Read the model definition and answer for the solid it produces. Units are mm, in the model's axes. A direction names the side the tool comes from. Coordinates: 2 decimals unless noted, no trailing zeros. Write each loop counter-clockwise with the first axis right and the second up, starting at its lowest first coordinate (ties: lowest second). Pieces come first, ordered by that corner, then holes.
(1) Straight lines are drawn through the part: line 1 along Y through (x, z) = (9, -5); line 2 along Z through (x, y) = (16.5, 0); line 3 along X through (y, z) = (-2.95, 0). For each, find the intervals that lie inside material, in ascending order.
(2) Determine the mould class of faces 5 (the cylindrical face through (10.074, -5.014, 0.404)), 6 (the cylindrical face through (14.79, 1.23, 6.14)), 7 (the flat face through (15, 6, 0)) for opening direction Y: pulls with the +Y half, pulls with the -Y half, needs draft (parallel to the pull), parting line crosses it, or undercut.
(3) The part is cut by section D-D, the plane z = -10.05. Determine the outline of the cut face in (x, y).
(4) The part is cut by section B-B, the plane y = 0. Determine the outline of the cut face in (x, z).
(5) The part is cut by section C-C, the plane x = 7. Determine the outline of the cut face in (y, z), and give its area (3 significant figures).
(6) Which of the six approach directions +Z, -Z, +X, -X, +Y, -Y give full straight-line access (tool end or side, diameter ignored) to faces 1 (the flat face through (20, -12, 14.15)), 2 (the flat face through (24, -14, 15)), 3 (the flat face through (9, 1, 0)), 4 (the flat face through (5.7, -4, -1.3))?
(7) The part is cut by section A-A, the plane z = 0. Determine the outline of the cut face in (x, y), and give its area (3 significant figures).
(8) Given pin 1 (6 mm diameter, centred on x = 4, z = 4, fed in from -Y); pin 2 (1 mm diameter, centred on y = 0, z = -15, fed in from -X); pin 3 (3 mm diameter, centred on x = 6.5, z = 1, fed in from -Y), each flat-ended and moving along its own axis, determine where each tip first touches the part or whether it passes through.
```python
from build123d import *

# Parameters (mm, degrees)
CROQUIS1_W              = 32.1
CROQUIS1_H              = 12
CROQUIS1_R              = 4.1
SALIENTE_EXTRUIR1_DEPTH = 30
CROQUIS2_W              = 15
CROQUIS2_H              = 2
CORTAR_EXTRUIR2_DEPTH   = 33
CROQUIS4_R              = 1.65
CORTAR_EXTRUIR3_DEPTH   = 12
CROQUIS5_R              = 3.1
CORTAR_EXTRUIR4_DEPTH   = 2
SALIENTE_EXTRUIR2_DEPTH = 16
REDONDEO1_R             = 5
REDONDEO2_R             = 5
REDONDEO3_RADIUS        = 4.002255821
REDONDEO3_LENGTH        = 1.9


with BuildPart() as part:
    # Croquis1 → Saliente-Extruir1 (new body)
    with BuildSketch(Plane(origin=(0, 0, 0), x_dir=(0, 0, -1), z_dir=(1, 0, 0))):
        Rectangle(CROQUIS1_W, CROQUIS1_H)
        with Locations((-10.05, 0)):
            Circle(CROQUIS1_R, mode=Mode.SUBTRACT)
        with Locations((10.05, 0)):
            Circle(CROQUIS1_R, mode=Mode.SUBTRACT)
    extrude(amount=SALIENTE_EXTRUIR1_DEPTH)

    # Croquis2 → Cortar-Extruir2 (cut)
    with BuildSketch(Plane.XY.offset(16.05)):
        with Locations((7.5, 0)):
            Rectangle(CROQUIS2_W, CROQUIS2_H)
    extrude(amount=-CORTAR_EXTRUIR2_DEPTH, mode=Mode.SUBTRACT)

    # Croquis4 → Cortar-Extruir3 (cut)
    with BuildSketch(Plane(origin=(0, 6, 0), x_dir=(1, 0, 0), z_dir=(0, 1, 0))):
        with Locations(Location((7, 0, 0), (0, 0, 270))):
            Circle(CROQUIS4_R)
    extrude(amount=-CORTAR_EXTRUIR3_DEPTH, mode=Mode.SUBTRACT)

    # Croquis5 → Cortar-Extruir4 (cut)
    with BuildSketch(Plane.XZ.offset(6)):
        with Locations(Location((7, 0, 0), (0, 0, 270))):
            Circle(CROQUIS5_R)
    extrude(amount=-CORTAR_EXTRUIR4_DEPTH, mode=Mode.SUBTRACT)

    # Croquis7 → Saliente-Extruir2 (add)
    with BuildSketch(Plane.XZ.offset(6)):
        Polygon((20, 14.15), (24, 14.15), (24, 16.05), (15.995488358, 16.05), (15.995488358, 14.15), align=None)
    extrude(amount=SALIENTE_EXTRUIR2_DEPTH)

    # Redondeo1
    redondeo1_edges = [part.edges().sort_by_distance(p)[0] for p in [
        (15.995488358, -6, 15.1),
    ]]
    fillet(redondeo1_edges, radius=REDONDEO1_R)

    # Redondeo2
    redondeo2_edges = [part.edges().sort_by_distance(p)[0] for p in [
        (24, -6, 15.1),
    ]]
    fillet(redondeo2_edges, radius=REDONDEO2_R)

    # Redondeo3: full round fillet: the end face becomes a half cylinder, R = half its width
    redondeo3_face = Plane((19.997744179, -22, 15.1), x_dir=(0, 0, 1), z_dir=(0, -1, 0))  # on the end face: x along it, z out of the body
    redondeo3_slab = redondeo3_face.offset(-REDONDEO3_RADIUS / 2) * Box(REDONDEO3_LENGTH, 2 * REDONDEO3_RADIUS, REDONDEO3_RADIUS, mode=Mode.PRIVATE)  # the body's end, R deep
    redondeo3_round = Plane((19.997744179, -17.997744179, 15.1), x_dir=(0, -1, 0), z_dir=(0, 0, 1)) * Cylinder(REDONDEO3_RADIUS, REDONDEO3_LENGTH, mode=Mode.PRIVATE)  # its axis R under the face
    add(redondeo3_slab - redondeo3_round, mode=Mode.SUBTRACT)


solid = part.part
```
Computed:
1. line 1: y = -6 to -1, 1 to 6
1. line 2: z = -16.05 to -14.15, -5.95 to 5.95, 14.15 to 16.05
1. line 3: x = 0 to 5.35, 8.65 to 30
2. face 5: needs draft
2. face 6: undercut
2. face 7: pulls with the +Y half
3. outline: (0, -6) - (30, -6) - (30, -4.1) - (0, -4.1) - close; (0, 4.1) - (30, 4.1) - (30, 6) - (0, 6) - close
4. outline: (15, -16.05) - (30, -16.05) - (30, -14.15) - (15, -14.15) - close; (15, -5.95) - (30, -5.95) - (30, 5.95) - (15, 5.95) - close; (15, 14.15) - (30, 14.15) - (30, 16.05) - (15, 16.05) - close
5. outline: (-6, -16.05) - (-1, -16.05) - (-1, -14.03) arc R4.1 cw to (-1, -6.07) - (-1, -1.65) - (-4, -1.65) - (-4, -3.1) - (-6, -3.1) - close; (-6, 3.1) - (-4, 3.1) - (-4, 1.65) - (-1, 1.65) - (-1, 6.07) arc R4.1 cw to (-1, 14.03) - (-1, 16.05) - (-6, 16.05) - close; (1, -16.05) - (6, -16.05) - (6, -1.65) - (1, -1.65) - (1, -6.07) arc R4.1 cw to (1, -14.03) - close; (1, 1.65) - (6, 1.65) - (6, 16.05) - (1, 16.05) - (1, 14.03) arc R4.1 cw to (1, 6.07) - close
5. area: 209 mm2
6. face 1: -Z, +X, -X, -Y
6. face 2: +Z, -Z, +X, -Y
6. face 3: +Z, -Z, -X
6. face 4: -Y
7. outline: (0, -6) - (3.9, -6) - (3.9, -4) - (5.35, -4) - (5.35, -1) - (0, -1) - close; (0, 1) - (5.35, 1) - (5.35, 6) - (0, 6) - close; (8.65, -4) - (10.1, -4) - (10.1, -6) - (30, -6) - (30, 6) - (8.65, 6) - (8.65, 1) - (15, 1) - (15, -1) - (8.65, -1) - close
7. area: 291 mm2
8. pin 1: stops at y = -6
8. pin 2: stops at x = 15
8. pin 3: stops at y = -4
